Geometry: see drawing. Coordinates: mm, zero at the bounding-box minimum. Round coordinates to 2 decimals unless told otherwise and drop trailing zeros. Order: outer loops, then holes, each group sorted by start corner. A loop starts at its lowest first (then second) coordinate and runs counter-clockwise, first axis right, second up. Notation, with made-up numbers: (48.5, -34.75) -> (58.5, -34.75) arc R31 cw to (58.5, -5.75) -> close; hole circle Ø11 at (-33, 26). An arc over 180 degrees is marked (long way). One line per item, written item: value. Start each with the question number.
1) Section C-C (y = 62). Return the cut outline in (x, z), and give its area (3 significant figures).
2) Section A-A (x = 68.5). Return the cut outline in (y, z).
3) Ray query, L1, parallel to Z at x = 3, y = 49. Return the intervals inside material, ascending.
4) Section B-B (z = 7). Return the cut outline in (x, y).
5) Section D-D (x = 55). Return the cut outline in (y, z).
6) Pin query (flat end, axial travel): P1, Ø6, axis at x = 49.5, y = 15, coming from the -Z side. Return the tip coordinate at first contact, or that it passes through.
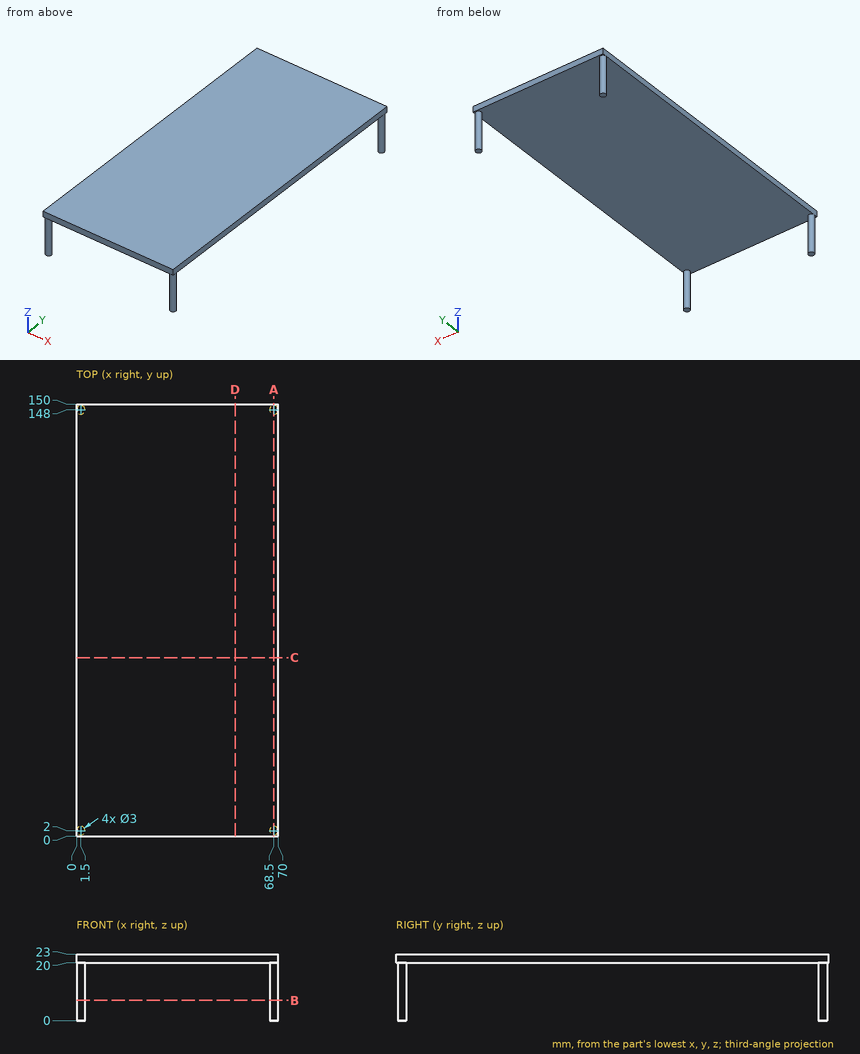
Findings:
1. outline: (0, 20) -> (70, 20) -> (70, 23) -> (0, 23) -> close
1. area: 210 mm2
2. outline: (0, 20) -> (0.5, 20) -> (0.5, 0) -> (3.5, 0) -> (3.5, 20) -> (146.5, 20) -> (146.5, 0) -> (149.5, 0) -> (149.5, 20) -> (150, 20) -> (150, 23) -> (0, 23) -> close
3. L1: 20 to 23
4. outline: circle Ø3 at (1.5, 2); circle Ø3 at (1.5, 148); circle Ø3 at (68.5, 2); circle Ø3 at (68.5, 148)
5. outline: (0, 20) -> (150, 20) -> (150, 23) -> (0, 23) -> close
6. P1: z = 20
